```python
from build123d import *

# Parameters (mm, degrees)
F0_R     = 12.1666
F1_DEPTH = 12.446
F0_R_2   = 31.75
F0_R_3   = 2.5781
F2_DEPTH = 4.572


with BuildPart() as f1:
    # F0 (on Front) → F1 (new body)
    with BuildSketch(Plane.XZ):
        Circle(F0_R)
        with BuildLine():
            ThreePointArc((3.30966, 3.77825), (5.02285, 0), (3.30966, -3.77825))
            Line((3.30966, -3.77825), (-3.30966, -3.77825))
            ThreePointArc((-3.30966, -3.77825), (-5.02285, 0), (-3.30966, 3.77825))
            Line((-3.30966, 3.77825), (3.30966, 3.77825))
        make_face(mode=Mode.SUBTRACT)
    extrude(amount=F1_DEPTH)

    # F0 (on Front) → F2 (join)
    with BuildSketch(Plane.XZ):
        Circle(F0_R_2)
        with Locations((-11.844468, -20.0771)):
            Circle(F0_R_3, mode=Mode.SUBTRACT)
        with Locations((11.465044, -20.29616)):
            Circle(F0_R_3, mode=Mode.SUBTRACT)
        with Locations((23.309512, -0.21906)):
            Circle(F0_R_3, mode=Mode.SUBTRACT)
        with Locations((-23.309512, 0.21906)):
            Circle(F0_R_3, mode=Mode.SUBTRACT)
        with Locations((-11.465044, 20.29616)):
            Circle(F0_R_3, mode=Mode.SUBTRACT)
        Circle(F0_R, mode=Mode.SUBTRACT)
        with Locations((11.844468, 20.0771)):
            Circle(F0_R_3, mode=Mode.SUBTRACT)
    extrude(amount=F2_DEPTH)


solid = f1.part
```
Verification items for the finished model (mm, model axes). A direction names the side the tool comes from. Round coordinates to 2 decimals unless told otherwise and drop trailing zeros. Order: outer loops, then holes, each group sorted by start corner. A loop starts at its lowest first (then second) coordinate and runs counter-clockwise, first axis right, second up. Notation, with made-up numbers: (57, -29.75) - (115, -29.75) arc R29 ccw to (115, -7.75) - close; hole circle Ø10 at (-38.75, 27.25). An arc over 180 degrees is marked (long way). Use CSV: the item, a comma, the result in double quotes.
(1) Section check A-A on x = 0. Record the boundary of the cut face in (y, z), and give its area (3 significant figures).
Entries:
outline,"(-12.45, -12.17) - (-4.57, -12.17) - (-4.57, -31.75) - (0, -31.75) - (0, -3.78) - (-12.45, -3.78) - close; (-12.45, 3.78) - (0, 3.78) - (0, 31.75) - (-4.57, 31.75) - (-4.57, 12.17) - (-12.45, 12.17) - close"
area,"388 mm^2"
(2) Section check B-B on y = -10.75. Record the boundary of the cut face in (x, z).
Entries:
outline,"circle Ø24.33 at (0, 0); hole (-3.31, -3.78) - (3.31, -3.78) arc R5.02 ccw to (3.31, 3.78) - (-3.31, 3.78) arc R5.02 ccw to start"
(3) Mould release check, pull along Z, two halves, no side actions. Record for faces 4 (the face through (0, 0, -7)), 5 (the face through (-9.084, -2.254, 19.309)), 6 (the face through (-6.883, -2.254, -30.995)): released by +Z, released by -Z, zero draft, split by the parting line, or undercut.
Entries:
face 4,"zero draft"
face 5,"undercut"
face 6,"split by the parting line"
(4) Gauge pin test, flat ends, axial feed: pin 1 Ø2 at (y, z) = (-6, -9.5) entering from +X; pin 2 Ø5.5 at (x, y) = (0.5, -3) entering from +Z; pin 3 Ø1 at (x, y) = (-20.5, -2) entering from +Z. Record the tip position at first contact, or that the pin passes through.
Entries:
pin 1,"x = 8.7"
pin 2,"z = 31.75"
pin 3,"z = 24.66"
(5) Access from +Z, -Z, +X, -X, +Y, -Y to the whole of each face (thin tool, end or side, straight path). Record for faces 1 (the face through (0, -4.572, -14)), 2 (the face through (0, -6, 3.778)), 3 (the face through (0, -12.446, -5)).
Entries:
face 1,"-Y"
face 2,"+Y, -Y"
face 3,"+Z, -Z, +X, -X, -Y"
(6) Thickness scan on probe 1 along X at (y, z) = (-1, 20); probe 2 along Z at (x, y) = (13.5, -4.25); probe 3 along Y at (x, z) = (18, 5). Record the ranges inside material, lowest first. Write a range as from..to.
Entries:
probe 1,"-24.66..-14.03, -8.9..9.27, 14.42..24.66"
probe 2,"-28.74..-21.88, -18.71..18.1, 22.05..28.74"
probe 3,"-4.57..0"
(7) Section check D-D on x = 25. Record the boundary of the cut face in (y, z), and give its area (3 significant figures).
Entries:
outline,"(-4.57, -19.57) - (0, -19.57) - (0, -2.17) - (-4.57, -2.17) - close; (-4.57, 1.73) - (0, 1.73) - (0, 19.57) - (-4.57, 19.57) - close"
area,"161 mm^2"
(8) Section check C-C on z = 10. Record the boundary of the cut face in (x, y), and give its area (3 significant figures).
Entries:
outline,"(-30.13, -4.57) - (-6.93, -4.57) - (-6.93, -12.45) - (6.93, -12.45) - (6.93, -4.57) - (30.13, -4.57) - (30.13, 0) - (-30.13, 0) - close"
area,"385 mm^2"
